Check sheet for the modelled part. Datum: model origin and axes. Units: mm. Face numbers are marked on the shaded views. A direction names the side the tool comes from. Give positions to 0.01 mm unless a question says otherwise; leave off trailing zeros. Order: outer loops, then holes, each group sorted by start corner. A loop starts at its lowest first (then second) coordinate and runs counter-clockwise, first axis right, second up. Notation, with made-up numbers: (-8, 55) - (20, 55) arc R22 ccw to (20, 84) - close; hole circle Ø10 at (44.5, -9.5). An arc over 180 degrees is marked (long way). Answer in a Markdown table with one row per item.
from build123d import *

# Parameters (mm, degrees)
SKETCH2_R           = 4.15
CUT_EXTRUDE1_DEPTH  = 26.999999876
BOSS_EXTRUDE1_DEPTH = 12
SKETCH4_R           = 4.62499994
CUT_EXTRUDE2_DEPTH  = 10.62
SKETCH5_R           = 2
CUT_EXTRUDE3_DEPTH  = 22.86
BOSS_EXTRUDE2_DEPTH = 2
SKETCH7_W           = 15.24
SKETCH7_H           = 13.999999876
CUT_EXTRUDE4_DEPTH  = 12.699999968


with BuildPart() as part:
    # Sketch1 → Revolve1 (revolve)
    with BuildSketch(Plane.XY):
        Polygon((0, 0), (-14.000000152, 0), (-14.000000152, 11.999999876), (-20.500000052, 11.999999876), (-20.500000052, 25.999999876), (-17.500000052, 25.999999876), (-17.500000052, 14.999999876), (-11.000000152, 14.999999876), (-11.000000152, 6.999999906), (0, 6.999999906), align=None)
    revolve(axis=Axis((0, 6.999999906, 0), (0, -1, 0)))

    # Sketch2 → Cut-Extrude1 (cut, through all)
    with BuildSketch(Plane.XZ):
        Circle(SKETCH2_R)
    extrude(amount=-CUT_EXTRUDE1_DEPTH, mode=Mode.SUBTRACT)

    # Sketch3 → Boss-Extrude1 (add)
    with BuildSketch(Plane.XZ.offset(-11.999999876)):
        with BuildLine():
            Line((-14.000000152, 0), (-14.000000152, -25.4))
            Line((-14.000000152, -25.4), (14.000000152, -25.4))
            Line((14.000000152, -25.4), (14.000000152, 0))
            ThreePointArc((14.000000152, 0), (0, -14.000000152), (-14.000000152, 0))
        make_face()
    extrude(amount=BOSS_EXTRUDE1_DEPTH)

    # Sketch4 → Cut-Extrude2 (cut)
    with BuildSketch(Plane.XZ):
        with Locations((0, -18.1)):
            Circle(SKETCH4_R)
    extrude(amount=-CUT_EXTRUDE2_DEPTH, mode=Mode.SUBTRACT)

    # Sketch5 → Cut-Extrude3 (cut)
    with BuildSketch(Plane.ZY.offset(14.000000152)):
        with Locations((-18.1, 6.000000096)):
            Circle(SKETCH5_R)
    extrude(amount=-CUT_EXTRUDE3_DEPTH, mode=Mode.SUBTRACT)

    # Sketch6 → Boss-Extrude2 (add)
    with BuildSketch(Plane(origin=(0, 11.999999876, 0), x_dir=(1, 0, 0), z_dir=(0, 1, 0))):
        with BuildLine():
            Line((14.000000152, 14.974979061), (14.000000152, 25.4))
            Line((14.000000152, 25.4), (-14.000000152, 25.4))
            Line((-14.000000152, 25.4), (-14.000000152, 14.974979061))
            ThreePointArc((-14.000000152, 14.974979061), (0, 20.500000052), (14.000000152, 14.974979061))
        make_face()
    extrude(amount=BOSS_EXTRUDE2_DEPTH)

    # Sketch7 → Cut-Extrude4 (cut)
    with BuildSketch(Plane.ZY.offset(20.500000052)):
        with Locations((-17.78, 6.999999938)):
            Rectangle(SKETCH7_W, SKETCH7_H)
    cut_extrude4 = extrude(amount=-CUT_EXTRUDE4_DEPTH, mode=Mode.SUBTRACT)

    # Mirror1: Cut-Extrude4 across plane
    add(cut_extrude4.mirror(Plane(origin=(0, 0, 0), x_dir=(0, 0, 1), z_dir=(1, 0, 0))), mode=Mode.SUBTRACT)


solid = part.part
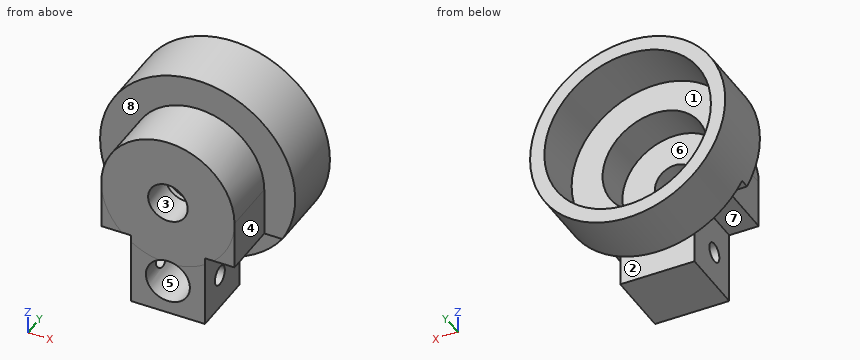
(1) Cross-section at A-A, the plane y = 6. Record the cut outline in (x, z) (3 decimals), then the cut area to 3 significant figures.
Geometry says:
| item | result |
|---|---|
| outline | (-14, -10.16) - (-7.8, -10.16) - (-7.8, -16.1) - (-4.17, -16.1) arc R4.625 cw to (4.17, -16.1) - (7.8, -16.1) - (7.8, -10.16) - (14, -10.16) - (14, 0) arc R14 ccw to (-14, 0) - close; (-7.8, -25.4) - (7.8, -25.4) - (7.8, -20.1) - (4.17, -20.1) arc R4.625 cw to (-4.17, -20.1) - (-7.8, -20.1) - close; hole circle Ø8.3 at (0, 0) |
| area | 682 mm² |
(2) Access from +Z, -Z, +X, -X, +Y, -Y to the whole of each face (thin tool, end or side, straight path). Record for the marked faces 5, 6, 7 and 8.
Geometry says:
| item | result |
|---|---|
| face 5 | -Y |
| face 6 | +Y |
| face 7 | -Z, -X, -Y |
| face 8 | +Z, -Y |
(3) Cross-section at C-C, the plane y = 9.5. Record the cut outline in (x, z) (3 decimals).
Geometry says:
| item | result |
|---|---|
| outline | (-14, -10.16) - (-7.8, -10.16) - (-7.8, -25.4) - (7.8, -25.4) - (7.8, -10.16) - (14, -10.16) - (14, 0) arc R14 ccw to (-14, 0) - close; hole circle Ø22 at (0, 0); hole circle Ø9.25 at (0, -18.1) |
(4) Mould release check, pull along X, two halves, no side actions. Record for the marked faces 1, 2, 3 and 4: pulls with the +X half, pulls with the -X half, needs draft (parallel to the pull), parting line crosses it, or undercut.
Geometry says:
| item | result |
|---|---|
| face 1 | undercut |
| face 2 | needs draft |
| face 3 | undercut |
| face 4 | pulls with the +X half |
(5) Thickness scan on L1, parallel to Z at x = 0, y = 7.5 (3 decimals); L2, parallel to Z at x = -2, y = 8.5; L3, parallel to X at y = 3.75, z = -18.1 (3 decimals). Record the ranges inside material, lowest first.
Geometry says:
| item | result |
|---|---|
| L1 | -25.4 to -22.725, -13.475 to -11, 11 to 14 |
| L2 | -25.4 to -22.27, -13.93 to -10.82, 10.82 to 13.86 |
| L3 | -7.8 to -4.625, 4.625 to 7.8 |
(6) Cross-section at D-D, the plane z = -18.1. Record the cut outline in (x, y) (3 decimals), then the cut area to 3 significant figures.
Geometry says:
| item | result |
|---|---|
| outline | (-9.625, 14) - (-7.8, 14) - (-7.8, 8) - (-4.625, 8) - (-4.625, 10.62) - (4.625, 10.62) - (4.625, 8) - (7.8, 8) - (7.8, 14) - (9.625, 14) - (9.625, 26) - (-9.625, 26) - close; (-7.8, 0) - (-4.625, 0) - (-4.625, 4) - (-7.8, 4) - close; (4.625, 0) - (7.8, 0) - (7.8, 4) - (4.625, 4) - close |
| area | 326 mm² |
(7) Gauge pin test, flat ends, axial feed: P1, Ø5, axis at y = 6, z = -18.1, coming from the +X side; P2, Ø1.9, axis at x = -0.5, z = -22, coming from the +Y side; P3, Ø4, axis at y = 7.5, z = -18, coming from the -X side; P4, Ø3, axis at y = 6, z = -18.1, coming from the +X side. Record the tip position at first contact, or that the pin passes through.
Geometry says:
| item | result |
|---|---|
| P1 | x = 7.8 |
| P2 | y = 14 |
| P3 | x = -7.8 |
| P4 | through |
(8) Cross-section at B-B, the plane x = 0. Record the cut outline in (y, z) (3 decimals).
Geometry says:
| item | result |
|---|---|
| outline | (0, -25.4) - (14, -25.4) - (14, -20.5) - (26, -20.5) - (26, -17.5) - (15, -17.5) - (15, -11) - (7, -11) - (7, -4.15) - (0, -4.15) - (0, -13.475) - (10.62, -13.475) - (10.62, -22.725) - (0, -22.725) - close; (0, 4.15) - (7, 4.15) - (7, 11) - (15, 11) - (15, 17.5) - (26, 17.5) - (26, 20.5) - (12, 20.5) - (12, 14) - (0, 14) - close |
